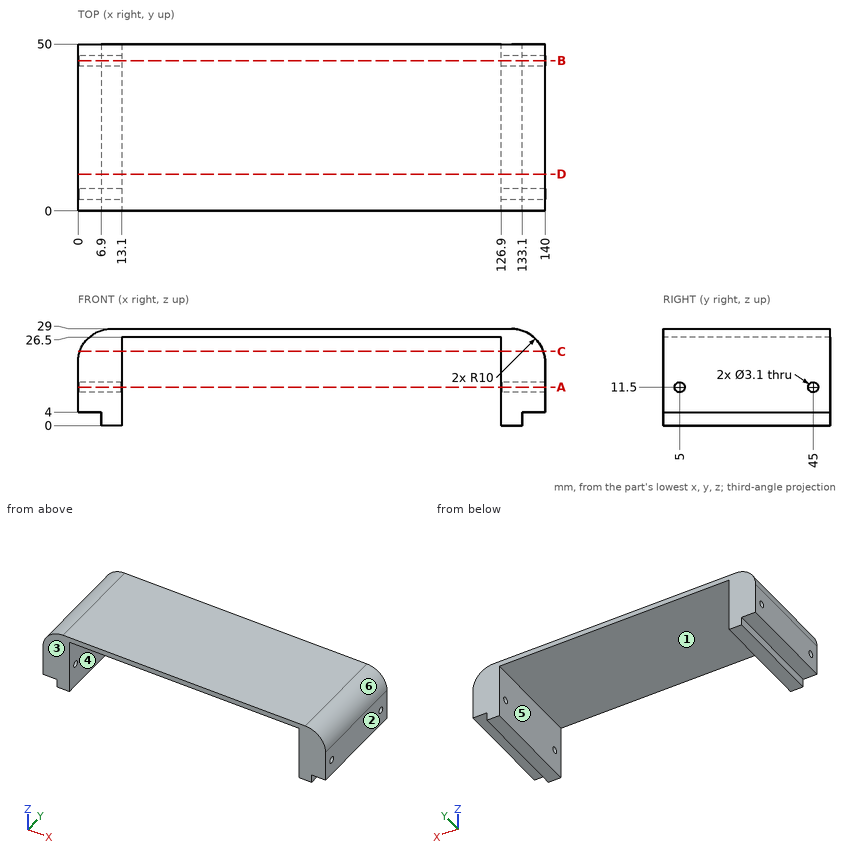
Design review of the part shown in the three views and the two pictorial views. Dimensions are in mm from the part's minimum x, y and z. A direction names the side the tool comes from. Round coordinates to 2 decimals unless told otherwise and drop trailing zeros. Order: outer loops, then holes, each group sorted by start corner. A loop starts at its lowest first (then second) coordinate and runs counter-clockwise, first axis right, second up. Notation, with made-up numbers: M 57.5,-11.5 L 93.5,-11.5 A31 ccw 93.5,16.5 Z; hole C 86,50.25 d11. An arc over 180 degrees is marked long. Put each result on its own line as item: value.
Q1. Machinability: for the marked faces 1 and 2, which of the approach directions +Z, -Z, +X, -X, +Y, -Y give a long, thin tool a straight path to every point of the face, cutting with its end or side? Answer none if there is none.
Reported:
face 1: -Z, +Y, -Y
face 2: +Z, -Z, +X, +Y, -Y
Q2. Consider section B-B (y = 45). State the section outline as (x, z) points, and give its area (3 significant figures).
Reported:
outline: M 0,4 L 6.9,4 L 6.9,0 L 13.1,0 L 13.1,9.95 L 0,9.95 Z; M 0,13.05 L 13.1,13.05 L 13.1,26.5 L 126.9,26.5 L 126.9,13.05 L 140,13.05 L 140,19 A10 ccw 130,29 L 10,29 A10 ccw 0,19 Z; M 126.9,0 L 133.1,0 L 133.1,4 L 140,4 L 140,9.95 L 126.9,9.95 Z
area: 865 mm²
Q3. Consider section A-A (z = 11.5). State the section outline as (x, y) points, and give its area (3 significant figures).
Reported:
outline: M 0,0 L 13.1,0 L 13.1,3.45 L 0,3.45 Z; M 0,6.55 L 13.1,6.55 L 13.1,43.45 L 0,43.45 Z; M 0,46.55 L 13.1,46.55 L 13.1,50 L 0,50 Z; M 126.9,0 L 140,0 L 140,3.45 L 126.9,3.45 Z; M 126.9,6.55 L 140,6.55 L 140,43.45 L 126.9,43.45 Z; M 126.9,46.55 L 140,46.55 L 140,50 L 126.9,50 Z
area: 1,150 mm²
Q4. Consider section C-C (z = 22.25). State the section outline as (x, y) points, and give its area (3 significant figures).
Reported:
outline: M 0.54,0 L 13.1,0 L 13.1,50 L 0.54,50 Z; M 126.9,0 L 139.46,0 L 139.46,50 L 126.9,50 Z
area: 1,260 mm²
Q5. Draft analysis for pull direction X (two halves, no side actions). For the marked faces 3, 4, 5 and 6, state which applies: released by +X, released by -X, zero draft, split by the parting line, or undercut.
Reported:
face 3: zero draft
face 4: undercut
face 5: undercut
face 6: released by +X
Q6. Consider section D-D (y = 11). State the section outline as (x, z) points, and give its area (3 significant figures).
Reported:
outline: M 0,4 L 6.9,4 L 6.9,0 L 13.1,0 L 13.1,26.5 L 126.9,26.5 L 126.9,0 L 133.1,0 L 133.1,4 L 140,4 L 140,19 A10 ccw 130,29 L 10,29 A10 ccw 0,19 Z
area: 946 mm²
Q7. Insertion check: pin 1 Ø1.5 at (x, y) = (66, 32) entering from -Z; pin 2 Ø3.5 at (x, y) = (4, 26.5) entering from -Z; pin 3 Ø2.5 at (y, z) = (45, 11.5) entering from -X; pin 4 Ø2 at (y, z) = (22.5, 2.5) entering from +X. Each pin has a flat end and moves straight along its axis. Give the tip position at first contact, or say it passes through.
Reported:
pin 1: z = 26.5
pin 2: z = 4
pin 3: through
pin 4: x = 133.1
Q8. To check wall thickness, follow line 1 (X direction, y = 21.5, z = 17.5); line 2 (Z direction, x = 115, y = 42.5); line 3 (X direction, y = 40, z = 22.5). State the ranges of each line that lie inside material, in increasing order.
Reported:
line 1: 0 to 13.1, 126.9 to 140
line 2: 26.5 to 29
line 3: 0.63 to 13.1, 126.9 to 139.37
